from build123d import *

# Parameters (mm, degrees)
F0_W     = 200
F0_H     = 200
F1_DEPTH = 10
F2_W     = 10
F2_H     = 110
F2_W_2   = 145
F2_H_2   = 10
F3_DEPTH = 6
F6_D     = 50
F7_W     = 50
F7_H     = 10
F8_DEPTH = 10
F10_D    = 8
F11_R    = 25


with BuildPart() as f1:
    # F0 (on Right) → F1 (new body)
    with BuildSketch(Plane.YZ):
        with Locations((100, 100)):
            Rectangle(F0_W, F0_H)
    extrude(amount=F1_DEPTH)

    # F2 (on face) → F3 (cut)
    with BuildSketch(Plane.YZ.offset(10)):
        Polygon((113.66365, 164.129353), (7.41181, 135.659258), (10, 126), (116.251841, 154.470095), align=None)
        Polygon((97.804037, 186.82684), (93.075355, 178.015508), (190, 126), (194.728683, 134.811331), align=None)
        with Locations((20, 70)):
            Rectangle(F2_W, F2_H)
        with Locations((100, 20)):
            Rectangle(F2_W_2, F2_H_2)
        with Locations((180, 70)):
            Rectangle(F2_W, F2_H)
    extrude(amount=-F3_DEPTH, mode=Mode.SUBTRACT)

    # F6 (through all)
    with Locations(Plane(origin=(0, 0, 0), x_dir=(0, -1, 0), z_dir=(-1, 0, 0))):
        with Locations((-100, 110)):
            Hole(F6_D / 2)

    # F7 (on face) → F8 (cut, through all)
    with BuildSketch(Plane(origin=(0, 0, 0), x_dir=(0, -1, 0), z_dir=(-1, 0, 0))):
        with Locations((-100, 65)):
            Rectangle(F7_W, F7_H)
    extrude(amount=-F8_DEPTH, mode=Mode.SUBTRACT)

    # F10 (through all)
    with Locations(Plane(origin=(0, 0, 0), x_dir=(0, -1, 0), z_dir=(-1, 0, 0))):
        with Locations((-150, 192), (-192, 150), (-50, 192), (-8, 150), (-50, 8), (-8, 50), (-150, 8), (-192, 50)):
            Hole(F10_D / 2)

    # F11
    f11_edges = [f1.edges().sort_by_distance(p)[0] for p in [
        (5, 0, 200),
        (5, 0, 0),
        (5, 200, 200),
        (5, 200, 0),
    ]]
    fillet(f11_edges, radius=F11_R)


solid = f1.part
Could you check a few things on this model? Use its own coordinates, in mm. A direction names the side the tool comes from. Give positions to 0.01 mm unless a question says otherwise; leave off trailing zeros. Order: outer loops, then holes, each group sorted by start corner. A loop starts at its lowest first (then second) coordinate and runs counter-clockwise, first axis right, second up. Notation, with made-up numbers: (22.25, 18.5) - (62.25, 18.5) arc R8 ccw to (62.25, 33.5) - close; hole circle Ø6 at (59.25, 89). An arc over 180 degrees is marked (long way). One line per question, with ' | ' between items. Start each with the question number.
Item 1: For faces 1 (the flat face through (5, 75, 65)), 2 (the flat face through (7, 180, 125)), 3 (the flat face through (5, 99, 0)), which set-ups out of +Z, -Z, +X, -X, +Y, -Y let a thin tool reach every point of the face, with its end or its side?
Item 2: I want a section at B-B on z = 50. Write out the boundary of the cut face in (x, y).
Item 3: I want a section at A-A on z = 110. Write out the boundary of the cut face in (x, y).
Item 4: I want a section at C-C on y = 178.5. Write out the boundary of the cut face in (x, z), then the cut area to 3 significant figures.
Item 5: I need wall thicknesses on probe 1 along Z at (x, y) = (5, 192); probe 2 along Z at (x, y) = (3, 48); probe 3 along Y at (x, z) = (4.25, 121). Which ranges of each line are inside material? Lowest first, please. Write a range as [from, to].
Item 6: Thinking about a two-plate mould opening in Y: for faces 4 (the flat face through (5, 99, 200)), 5 (the cylindrical face through (5.07, 195.815, 51.201)), 6 (the cylindrical face through (5.07, 7.129, 7.518)), 7 (the cylindrical face through (5.07, 192.482, 192.871)), which applies, pulls with the +Y half, pulls with the -Y half, needs draft (parallel to the pull), parting line crosses it, or undercut?
Item 7: I want a section at D-D on x = 6.75. Give the number of separate pieces and of enclosed holes in the cut face, then the cut area to 3 significant figures.
Item 8: I'm going to push a flat-ended pin straight in: pin 1 Ø1.8 at (x, y) = (5.5, 181) entering from +Z. Where does the tip first touch, or does it pass through?
Verdict:
1) face 1: +X, -X | face 2: +X | face 3: -Z, +X, -X, +Y, -Y
2) outline: (0, 0) - (10, 0) - (10, 4) - (0, 4) - close; (0, 12) - (10, 12) - (10, 15) - (4, 15) - (4, 25) - (10, 25) - (10, 175) - (4, 175) - (4, 185) - (10, 185) - (10, 188) - (0, 188) - close; (0, 196) - (10, 196) - (10, 200) - (0, 200) - close
3) outline: (0, 0) - (10, 0) - (10, 15) - (4, 15) - (4, 25) - (10, 25) - (10, 75) - (0, 75) - close; (0, 125) - (10, 125) - (10, 175) - (4, 175) - (4, 185) - (10, 185) - (10, 200) - (0, 200) - close
4) outline: (0, 0.25) - (10, 0.25) - (10, 15) - (4, 15) - (4, 125) - (10, 125) - (10, 132.17) - (4, 132.17) - (4, 143.52) - (10, 143.52) - (10, 199.75) - (0, 199.75) - close | area: 1,270 mm^2
5) probe 1: [6.67, 46], [54, 129.73], [136.28, 146], [154, 193.33] | probe 2: [0, 4.54], [11.46, 188.54], [195.46, 200] | probe 3: [0, 15], [25, 77.55], [122.45, 175], [185, 200]
6) face 4: needs draft | face 5: undercut | face 6: pulls with the -Y half | face 7: pulls with the +Y half
7) separate pieces: 1 | enclosed holes: 15 | area: 30,700 mm^2
8) pin 1: z = 199.47
